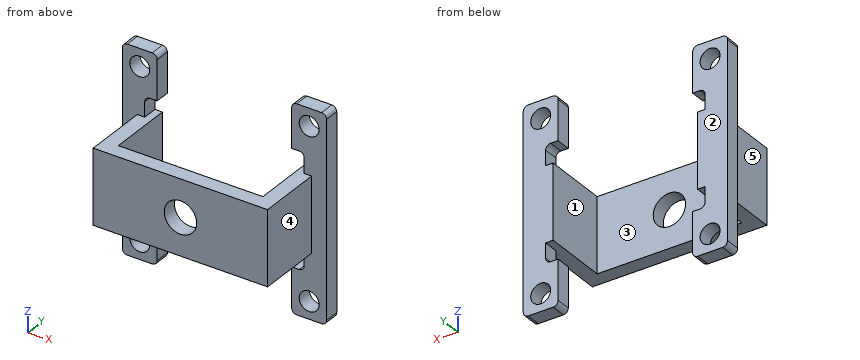
from build123d import *

# Parameters (mm, degrees)
SKETCH_1_R      = 3.25
EXTRUDE_1_DEPTH = 3
SKETCH_2_W      = 3
SKETCH_2_H      = 15
EXTRUDE_2_DEPTH = 10
SKETCH_3_R      = 2
EXTRUDE_3_DEPTH = 3


with BuildPart() as part:
    # 草图1 → 凸台-拉伸1 (new body)
    with BuildSketch(Plane(origin=(0, 0, 0), x_dir=(1, 0, 0), z_dir=(0, 1, 0))):
        Polygon((-12.5, 7.5), (12.5, 7.5), (17.5, 7.5), (17.5, -7.5), (12.5, -7.5), (-12.5, -7.5), (-17.5, -7.5), (-17.5, 7.5), align=None)
        with Locations(Location((0, 0, 0), (0, 0, 270))):
            Circle(SKETCH_1_R, mode=Mode.SUBTRACT)
    extrude(amount=EXTRUDE_1_DEPTH)

    # 草图2 → 凸台-拉伸2 (add)
    with BuildSketch(Plane(origin=(0, 3, 0), x_dir=(1, 0, 0), z_dir=(0, 1, 0))):
        with Locations((-16, 0)):
            Rectangle(SKETCH_2_W, SKETCH_2_H)
        with Locations((16, 0)):
            Rectangle(SKETCH_2_W, SKETCH_2_H)
    extrude(amount=EXTRUDE_2_DEPTH)

    # 草图3 → 凸台-拉伸3 (add)
    # profile 1 of 2: a face of its own
    with BuildSketch(Plane(origin=(0, 13, 0), x_dir=(1, 0, 0), z_dir=(0, 1, 0))):
        with BuildLine():
            Line((-15, -11.5), (-13.5, -11.5))
            Line((-13.5, -11.5), (-13.5, -17.5))
            Line((-13.5, -17.5), (-13.5, -19.5))
            ThreePointArc((-13.5, -19.5), (-13.792893219, -20.207106781), (-14.5, -20.5))
            Line((-14.5, -20.5), (-19.5, -20.5))
            ThreePointArc((-19.5, -20.5), (-20.207106781, -20.207106781), (-20.5, -19.5))
            Line((-20.5, -19.5), (-20.5, 19.5))
            ThreePointArc((-20.5, 19.5), (-20.207106781, 20.207106781), (-19.5, 20.5))
            Line((-19.5, 20.5), (-14.5, 20.5))
            ThreePointArc((-14.5, 20.5), (-13.792893219, 20.207106781), (-13.5, 19.5))
            Line((-13.5, 19.5), (-13.5, 18.5))
            Line((-13.5, 18.5), (-13.5, 11.5))
            Line((-13.5, 11.5), (-15, 11.5))
            ThreePointArc((-15, 11.5), (-15.707106781, 11.207106781), (-16, 10.5))
            Line((-16, 10.5), (-16, 7.5))
            Line((-16, 7.5), (-14.5, 7.5))
            Line((-14.5, 7.5), (-14.5, -7.5))
            Line((-14.5, -7.5), (-16, -7.5))
            Line((-16, -7.5), (-16, -10.5))
            ThreePointArc((-16, -10.5), (-15.707106781, -11.207106781), (-15, -11.5))
        make_face()
        with Locations(Location((-17, 17, 0), (0, 0, 270))):
            Circle(SKETCH_3_R, mode=Mode.SUBTRACT)
        with Locations(Location((-17, -17, 0), (0, 0, 90))):
            Circle(SKETCH_3_R, mode=Mode.SUBTRACT)
    # profile 2 of 2: a face of its own
    with BuildSketch(Plane(origin=(0, 13, 0), x_dir=(1, 0, 0), z_dir=(0, 1, 0))):
        with BuildLine():
            Line((14.5, 7.5), (16, 7.5))
            Line((16, 7.5), (16, 10.5))
            ThreePointArc((16, 10.5), (15.707106781, 11.207106781), (15, 11.5))
            Line((15, 11.5), (13.5, 11.5))
            Line((13.5, 11.5), (13.5, 18.5))
            Line((13.5, 18.5), (13.5, 19.5))
            ThreePointArc((13.5, 19.5), (13.792893219, 20.207106781), (14.5, 20.5))
            Line((14.5, 20.5), (19.5, 20.5))
            ThreePointArc((19.5, 20.5), (20.207106781, 20.207106781), (20.5, 19.5))
            Line((20.5, 19.5), (20.5, -19.5))
            ThreePointArc((20.5, -19.5), (20.207106781, -20.207106781), (19.5, -20.5))
            Line((19.5, -20.5), (14.5, -20.5))
            ThreePointArc((14.5, -20.5), (13.792893219, -20.207106781), (13.5, -19.5))
            Line((13.5, -19.5), (13.5, -18.5))
            Line((13.5, -18.5), (13.5, -11.5))
            Line((13.5, -11.5), (15, -11.5))
            ThreePointArc((15, -11.5), (15.707106781, -11.207106781), (16, -10.5))
            Line((16, -10.5), (16, -7.5))
            Line((16, -7.5), (14.5, -7.5))
            Line((14.5, -7.5), (14.5, 7.5))
        make_face()
        with Locations(Location((17, 17, 0), (0, 0, 90))):
            Circle(SKETCH_3_R, mode=Mode.SUBTRACT)
        with Locations(Location((17, -17, 0), (0, 0, 270))):
            Circle(SKETCH_3_R, mode=Mode.SUBTRACT)
    extrude(amount=EXTRUDE_3_DEPTH)


solid = part.part
Geometry: final body of the model. Coordinates: model frame, mm. Face numbers are marked on the shaded views. A direction names the side the tool comes from. Give positions to 0.01 mm unless a question says otherwise; leave off trailing zeros. Write each loop counter-clockwise with the first axis right and the second up, starting at its lowest first coordinate (ties: lowest second). Pieces come first, ordered by that corner, then holes.
(1) Cut plane A-A, the plane z = -13. Return loops of the section in (x, y), then the cut area to 3 significant figures.
(2) Cut plane D-D, the plane x = -17. Return loops of the section in (y, z).
(3) Mould query, pull axis X, two halves, no side actions, for the marked faces 3, 4 and 5. Classes: released by +X, released by -X, zero draft, split by the parting line, or undercut.
(4) Cut plane C-C, the plane z = 17. Return loops of the section in (x, y).
(5) Ray query, line 1 (X direction, y = 14.6, z = 17); line 2 (X direction, y = 3.25, z = -0.5); line 3 (X direction, y = 1.4, z = 0). Return the intervals inside material, ascending.
(6) Access query for the marked faces 1 and 2. Directions: +Z, -Z, +X, -X, +Y, -Y. A direction counts if a zero-diameter tool reaches every point of the face in a straight line with its end or side. Return the directions, or none.
(7) First-contact query: P1, Ø6.5, axis at y = 7.5, z = -0.5, coming from the -X side; P2, Ø2.5, axis at x = -17, z = -17, coming from the -Y side; P3, Ø5, axis at x = 4, y = 4.5, coming from the +Z side; P4, Ø5, axis at x = -10, y = 4, coming from the -Z side. Flat tips, straight axial feed; report the tip coordinate or a pass-through.
(8) Cut plane B-B, the plane y = 3.75. Return loops of the section in (x, z), then the cut area to 3 significant figures.
Values follow:
1. outline: (-20.5, 13) - (-13.5, 13) - (-13.5, 16) - (-20.5, 16) - close; (13.5, 13) - (20.5, 13) - (20.5, 16) - (13.5, 16) - close
1. area: 42.0 mm2
2. outline: (0, -7.5) - (13, -7.5) - (13, -15) - (16, -15) - (16, 15) - (13, 15) - (13, 7.5) - (0, 7.5) - close; (13, -20.5) - (16, -20.5) - (16, -19) - (13, -19) - close; (13, 19) - (16, 19) - (16, 20.5) - (13, 20.5) - close
3. face 3: undercut
3. face 4: released by +X
3. face 5: released by -X
4. outline: (-20.5, 13) - (-19, 13) - (-19, 16) - (-20.5, 16) - close; (-15, 13) - (-13.5, 13) - (-13.5, 16) - (-15, 16) - close; (13.5, 13) - (15, 13) - (15, 16) - (13.5, 16) - close; (19, 13) - (20.5, 13) - (20.5, 16) - (19, 16) - close
5. line 1: x = -20.5 to -19, -15 to -13.5, 13.5 to 15, 19 to 20.5
5. line 2: x = -17.5 to -14.5, 14.5 to 17.5
5. line 3: x = -17.5 to -3.25, 3.25 to 17.5
6. face 1: +Y
6. face 2: +Z, -Z, +X, -X, +Y
7. P1: stops at x = -17.5
7. P2: passes through
7. P3: stops at z = 7.5
7. P4: stops at z = -7.5
8. outline: (-17.5, -7.5) - (-14.5, -7.5) - (-14.5, 7.5) - (-17.5, 7.5) - close; (14.5, -7.5) - (17.5, -7.5) - (17.5, 7.5) - (14.5, 7.5) - close
8. area: 90.0 mm2
